Part model, mm, in its own coordinate system. A direction names the side the tool comes from. Round coordinates to 2 decimals unless told otherwise and drop trailing zeros. Order: outer loops, then holes, each group sorted by start corner. A loop starts at its lowest first (then second) coordinate and runs counter-clockwise, first axis right, second up. Notation, with made-up numbers: M -34,79.25 L -14,79.25 A24 ccw -14,97.25 Z; hole C 30,47 d7. An arc over 180 degrees is marked long. Write each question's results on one line, items separated by ' | '. Start each with the question number.
1. Two-plate mould, pull along Z, no slides. Class faces 3 (the face through (-5.98, 6.48, -6.75)), 4 (the face through (0, 1, 3)), 5 (the face through (9.14, 6.52, -8.1)), 6 (the face through (6.19, 6.48, -6.18)): +Z half, -Z half, draft (parallel to the pull), parting line (faces both ways), or undercut.
2. Drop flat-ended pins along their axis: pin 1 Ø4.5 at (x, y) = (-5, 0) entering from -Z; pin 2 Ø3.5 at (x, z) = (-4.8, -6) entering from -Y. Give the stop position or say it passes through.
3. Which spindle directions (+Z, -Z, +X, -X, +Y, -Y) get a long thin tool onto all of the face, cutting with end or side? Do faces 1 (the face through (3.283, -0.541, 1.479)), 2 (the face through (0, 5, -6)). Say none if no direction does.
4. Band-saw the part on A-A, the plane y = 0. List the corners of the cut face in (x, z).
5. Band-saw the part on C-C, the plane x = 4.8. List the corners of the cut face in (y, z), then the cut area to 3 significant figures.
6. Probe L1, parallel to Y at x = 5, z = 0.75; L2, parallel to Z at x = -4.8, y = 6.9; L3, parallel to Z at x = 2, y = 1.25. List the from-to ranges inside material, lowest first. Write a range as [from, to].
7. Band-saw the part on B-B, the plane y = 5.5. List the corners of the cut face in (x, z), then the cut area to 3 significant figures.
8. Band-saw the part on D-D, the plane z = 2. List the corners of the cut face in (x, y).
```python
from build123d import *

# Parameters (mm, degrees)
SKETCH1_W           = 20
SKETCH1_H           = 10
SKETCH1_R           = 1.8
BOSS_EXTRUDE1_DEPTH = 3
SKETCH2_W           = 20
SKETCH2_H           = 12
SKETCH2_R           = 1.4
BOSS_EXTRUDE2_DEPTH = 3
FILLET1_R           = 3


with BuildPart() as part:
    # Sketch1 → Boss-Extrude1 (new body)
    with BuildSketch(Plane.XY):
        Rectangle(SKETCH1_W, SKETCH1_H)
        with Locations((-5, 0)):
            Circle(SKETCH1_R, mode=Mode.SUBTRACT)
        with Locations(Location((5, 0, 0), (0, 0, 180))):
            Circle(SKETCH1_R, mode=Mode.SUBTRACT)
    extrude(amount=BOSS_EXTRUDE1_DEPTH)

    # Sketch2 → Boss-Extrude2 (add)
    with BuildSketch(Plane(origin=(0, 5, 0), x_dir=(1, 0, 0), z_dir=(0, 1, 0))):
        with Locations((0, 3)):
            Rectangle(SKETCH2_W, SKETCH2_H)
        with Locations(Location((4.8, 6, 0), (0, 0, 270))):
            Circle(SKETCH2_R, mode=Mode.SUBTRACT)
        with Locations(Location((-4.8, 6, 0), (0, 0, 90))):
            Circle(SKETCH2_R, mode=Mode.SUBTRACT)
    extrude(amount=BOSS_EXTRUDE2_DEPTH)

    # Fillet1
    fillet1_edges = [part.edges().sort_by_distance(p)[0] for p in [
        (-10, 6.5, -9),
        (10, 6.5, -9),
        (0, 5, 0),
        (10, -5, 1.5),
        (-10, -5, 1.5),
    ]]
    fillet(fillet1_edges, radius=FILLET1_R)


solid = part.part
```
Solution:
1) face 3: undercut | face 4: +Z half | face 5: -Z half | face 6: undercut
2) pin 1: z = -0.01 | pin 2: y = 5
3) face 1: +Z, -Z | face 2: -Z, +X, -X, -Y
4) outline: M -10,0 L -6.8,0 L -6.8,3 L -10,3 Z; M -3.2,0 L 3.2,0 L 3.2,3 L -3.2,3 Z; M 6.8,0 L 10,0 L 10,3 L 6.8,3 Z
5) outline: M -5,0 L -1.79,0 L -1.79,3 L -5,3 Z; M 1.79,0 L 2,0 A3 cw 5,-3 L 5,-4.6 L 8,-4.6 L 8,3 L 1.79,3 Z; M 5,-9 L 8,-9 L 8,-7.4 L 5,-7.4 Z | area: 48.8 mm^2
6) L1: [-5, -1.8], [1.8, 8] | L2: [-9, -7.4], [-4.6, 3] | L3: [0, 3]
7) outline: M -10,-6 A3 ccw -7,-9 L 7,-9 A3 ccw 10,-6 L 10,3 L -10,3 Z; hole C -4.8,-6 d2.8; hole C 4.8,-6 d2.8 | area: 224 mm^2
8) outline: M -10,-2 A3 ccw -7,-5 L 7,-5 A3 ccw 10,-2 L 10,8 L -10,8 Z; hole C -5,0 d3.6; hole C 5,0 d3.6
